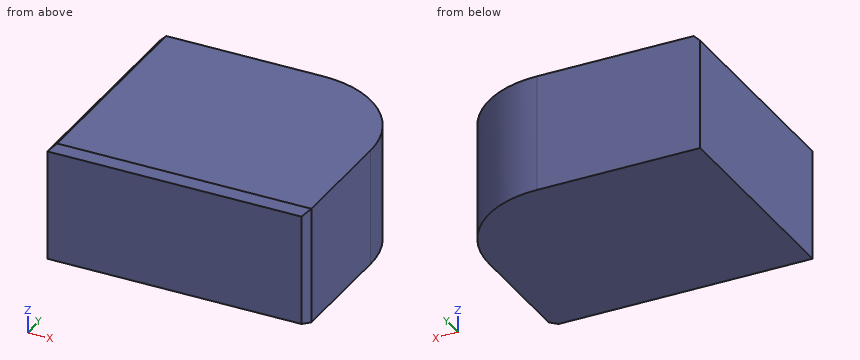
```python
from build123d import *

# Parameters (mm, degrees)
F0_W     = 204.106725
F0_H     = 172.404602
F1_DEPTH = 91.694
F2_SIZE  = 5.08
F3_R     = 76.2


with BuildPart() as f1:
    # F0 (on Top) → F1 (new body)
    with BuildSketch(Plane.XY):
        with Locations((29.834312, -9.587683)):
            Rectangle(F0_W, F0_H)
    extrude(amount=F1_DEPTH)

    # F2
    f2_edges = [f1.edges().sort_by_distance(p)[0] for p in [
        (29.834311, -95.789984, 91.694),
        (-72.219051, -9.587683, 91.694),
        (131.887674, -95.789984, 45.847),
    ]]
    chamfer(f2_edges, length=F2_SIZE)

    # F3
    f3_edges = [f1.edges().sort_by_distance(p)[0] for p in [
        (131.887674, 76.614618, 45.847),
    ]]
    fillet(f3_edges, radius=F3_R)


solid = f1.part
```
Verification items for the finished model (mm, model axes). Give positions to 0.01 mm unless a question says otherwise; leave off trailing zeros. Loops run counter-clockwise (first coordinate to the right, second up) from the corner with the lowest first, then second, coordinate; pieces in that order, holes last.
1. Section check B-B, the plane y = 45. Enter the section's corners in (x, z).
2. Section check A-A, the plane z = 29.5. Enter the section's corners in (x, y).
3. Thickness scan on line 1 (X direction, y = 34, z = 79.5); line 2 (X direction, y = 52, z = 5); line 3 (Y direction, x = 61, z = 57). Record the ranges inside material, lowest first.
4. Section check C-C, the plane x = 96. Enter the section's corners in (y, z), then the cut area to 3 significant figures.
Geometry says:
1. outline: (-72.22, 0) - (117.48, 0) - (117.48, 91.69) - (-67.14, 91.69) - (-72.22, 86.61) - close
2. outline: (-72.22, -95.79) - (126.81, -95.79) - (131.89, -90.71) - (131.89, 0.41) arc R76.2 ccw to (55.69, 76.61) - (-72.22, 76.61) - close
3. line 1: x = -72.22 to 124.09
3. line 2: x = -72.22 to 111.77
3. line 3: y = -95.79 to 76.43
4. outline: (-95.79, 0) - (65.08, 0) - (65.08, 91.69) - (-90.71, 91.69) - (-95.79, 86.61) - close
4. area: 14,700 mm2
